Can you work these out from the drawing? Everything is in mm from the part's minimum corner. Give positions to 0.01 mm unless a question says otherwise; leave off trailing zeros. Write each loop counter-clockwise with the first axis right and the second up, starting at its lowest first coordinate (ties: lowest second). Pieces come first, ordered by that corner, then holes. Notation, with made-up numbers: (55, -30.75) - (90, -30.75) arc R29 cw to (90, -2.75) - close; hole circle Ø8 at (72.25, -32). An arc over 180 degrees is marked (long way). Answer in a Markdown table with one row per item.
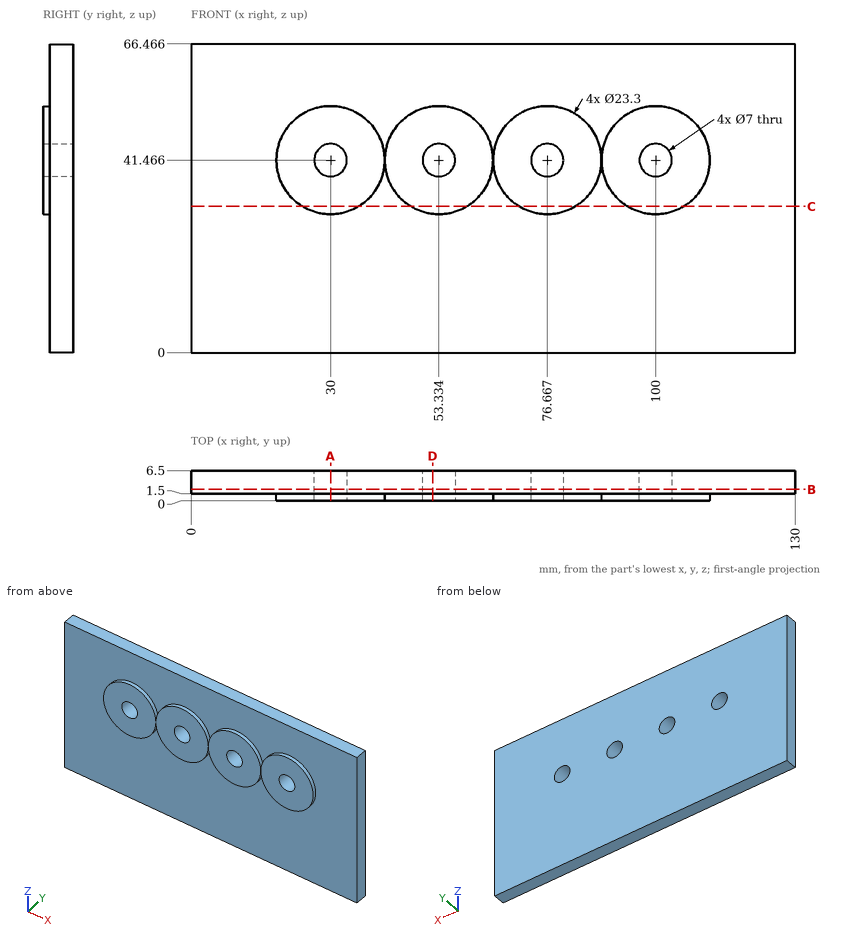
1) Imagine slicing it at D-D (x = 52). List the corners of the cut face in (y, z) for me (1 decimal), then the cut area to 3 significant figures.
Check values:
| item | result |
|---|---|
| outline | (0, 29.9) - (1.5, 29.9) - (1.5, 0) - (6.5, 0) - (6.5, 38.2) - (0, 38.2) - close; (0, 44.7) - (6.5, 44.7) - (6.5, 66.5) - (1.5, 66.5) - (1.5, 53) - (0, 53) - close |
| area | 325 mm2 |
2) Will these pins go through, and if not, where does the flat tip stop? P1, Ø9, axis at x = 100, z = 41.47, coming from the +Y side; P2, Ø3, axis at x = 114.5, z = 10, coming from the -Y side.
Check values:
| item | result |
|---|---|
| P1 | stops at y = 6.5 |
| P2 | stops at y = 1.5 |
3) If I drill on line 1 (Z direction, x = 30, y = 3.25) (1 decimal); line 2 (X direction, y = 6.25, z = 41) (1 decimal); line 3 (X direction, y = 6.25, z = 43) (1 decimal), over which ranges is the centre line in solid material (lowest first)?
Check values:
| item | result |
|---|---|
| line 1 | z = 0 to 38, 45 to 66.5 |
| line 2 | x = 0 to 26.5, 33.5 to 49.9, 56.8 to 73.2, 80.1 to 96.5, 103.5 to 130 |
| line 3 | x = 0 to 26.9, 33.1 to 50.2, 56.5 to 73.5, 79.8 to 96.9, 103.1 to 130 |
4) Imagine slicing it at B-B (y = 2.5). List the corners of the cut face in (x, z) for me (1 decimal), then the cut area to 3 significant figures.
Check values:
| item | result |
|---|---|
| outline | (0, 0) - (130, 0) - (130, 66.5) - (0, 66.5) - close; hole circle Ø7 at (30, 41.5); hole circle Ø7 at (53.3, 41.5); hole circle Ø7 at (76.7, 41.5); hole circle Ø7 at (100, 41.5) |
| area | 8,490 mm2 |
5) Imagine slicing it at A-A (x = 30). List the corners of the cut face in (y, z) for me (1 decimal), then the cut area to 3 significant figures.
Check values:
| item | result |
|---|---|
| outline | (0, 29.8) - (1.5, 29.8) - (1.5, 0) - (6.5, 0) - (6.5, 38) - (0, 38) - close; (0, 45) - (6.5, 45) - (6.5, 66.5) - (1.5, 66.5) - (1.5, 53.1) - (0, 53.1) - close |
| area | 322 mm2 |
6) Imagine slicing it at C-C (z = 31.5). List the corners of the cut face in (x, y) for me.
Check values:
| item | result |
|---|---|
| outline | (0, 1.5) - (23.97, 1.5) - (23.97, 0) - (36.03, 0) - (36.03, 1.5) - (47.3, 1.5) - (47.3, 0) - (59.37, 0) - (59.37, 1.5) - (70.63, 1.5) - (70.63, 0) - (82.7, 0) - (82.7, 1.5) - (93.97, 1.5) - (93.97, 0) - (106.03, 0) - (106.03, 1.5) - (130, 1.5) - (130, 6.5) - (0, 6.5) - close |
